```python
from build123d import *

# Parameters (mm, degrees)
SKETCH_1_W      = 64
SKETCH_1_H      = 13
SKETCH_1_R      = 2.75
SKETCH_1_R_2    = 1.6
EXTRUDE_1_DEPTH = 1.5
CHAMFER_1_SIZE  = 3.5
CHAMFER_2_SIZE  = 1.5


with BuildPart() as part:
    # 草图1 → 凸台-拉伸1 (new, symmetric)
    with BuildSketch(Plane.XY):
        Rectangle(SKETCH_1_W, SKETCH_1_H)
        with Locations((-25, 0)):
            Circle(SKETCH_1_R, mode=Mode.SUBTRACT)
        with Locations((25, 0)):
            Circle(SKETCH_1_R, mode=Mode.SUBTRACT)
        with Locations((-15, 0)):
            Circle(SKETCH_1_R_2, mode=Mode.SUBTRACT)
        with Locations(Location((15, 0, 0), (0, 0, 180))):
            Circle(SKETCH_1_R_2, mode=Mode.SUBTRACT)
    extrude(amount=EXTRUDE_1_DEPTH, both=True)

    # 倒角1
    chamfer_1_edges = [part.edges().sort_by_distance(p)[0] for p in [
        (32, -6.5, 0),
    ]]
    chamfer(chamfer_1_edges, length=CHAMFER_1_SIZE)

    # 倒角2
    chamfer_2_edges = [part.edges().sort_by_distance(p)[0] for p in [
        (-16.6, 0, 1.5),
        (16.6, 0, 1.5),
    ]]
    chamfer(chamfer_2_edges, length=CHAMFER_2_SIZE)


solid = part.part
```
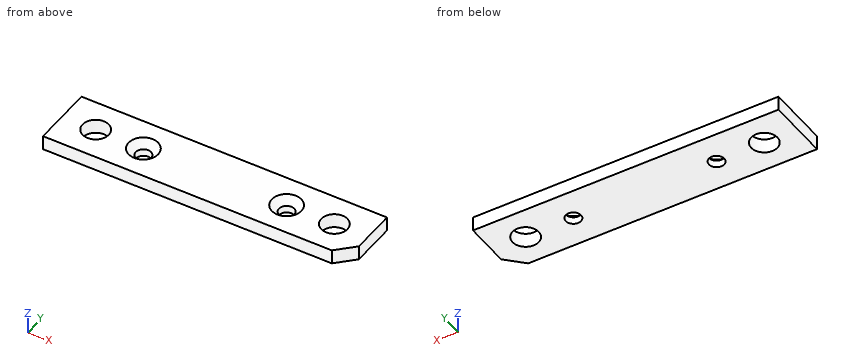
The listing builds one solid part. Answer for the finished solid, in the listing's coordinates (mm). Coordinates: 2 decimals unless noted, no trailing zeros. Write each loop counter-clockwise with the first axis right and the second up, starting at its lowest first coordinate (ties: lowest second). Pieces come first, ordered by that corner, then holes. Notation, with made-up numbers: (89.5, -3.5) - (122.5, -3.5) arc R13 cw to (122.5, 6.5) - close; hole circle Ø7 at (71.5, 68.25). An arc over 180 degrees is marked (long way). Return JSON: item names as keys, results as strings. Group by question number.
Q1. The part is cut by section B-B on z = 0.8. Write down the section's boundary in (x, y).
Q2. Find the intervals of material crossed by line 1 along Y through (x, z) = (25, -0.3); line 2 along X through (y, z) = (-1.25, 1); line 3 along X through (y, z) = (1.25, -0.9), in increasing order. Write a range as [from, to].
Q3. The part is cut by section A-A on x = -25. Write down the section's boundary in (y, z).
Q4. The part is cut by section D-D on x = 15. Write down the section's boundary in (y, z), and give its area (4 significant figures).
Q5. The part is cut by section C-C on y = 0. Write down the section's boundary in (x, z).
Evaluation:
{
 "1": {"outline": "(-32, -6.5) - (28.5, -6.5) - (32, -3) - (32, 6.5) - (-32, 6.5) - close; hole circle Ø5.5 at (-25, 0); hole circle Ø4.8 at (-15, 0); hole circle Ø4.8 at (15, 0); hole circle Ø5.5 at (25, 0)"},
 "2": {"line 1": "y = [-6.5, -2.75], [2.75, 6.5]", "line 2": "x = [-32, -27.45], [-22.55, -17.28], [-12.72, 12.72], [17.28, 22.55], [27.45, 32]", "line 3": "x = [-32, -27.45], [-22.55, -16], [-14, 14], [16, 22.55], [27.45, 32]"},
 "3": {"outline": "(-6.5, -1.5) - (-2.75, -1.5) - (-2.75, 1.5) - (-6.5, 1.5) - close; (2.75, -1.5) - (6.5, -1.5) - (6.5, 1.5) - (2.75, 1.5) - close"},
 "4": {"outline": "(-6.5, -1.5) - (-1.6, -1.5) - (-1.6, 0) - (-3.1, 1.5) - (-6.5, 1.5) - close; (1.6, -1.5) - (6.5, -1.5) - (6.5, 1.5) - (3.1, 1.5) - (1.6, 0) - close", "area": "27.15 mm2"},
 "5": {"outline": "(-32, -1.5) - (-27.75, -1.5) - (-27.75, 1.5) - (-32, 1.5) - close; (-22.25, -1.5) - (-16.6, -1.5) - (-16.6, 0) - (-18.1, 1.5) - (-22.25, 1.5) - close; (-13.4, -1.5) - (13.4, -1.5) - (13.4, 0) - (11.9, 1.5) - (-11.9, 1.5) - (-13.4, 0) - close; (16.6, -1.5) - (22.25, -1.5) - (22.25, 1.5) - (18.1, 1.5) - (16.6, 0) - close; (27.75, -1.5) - (32, -1.5) - (32, 1.5) - (27.75, 1.5) - close"}
}
